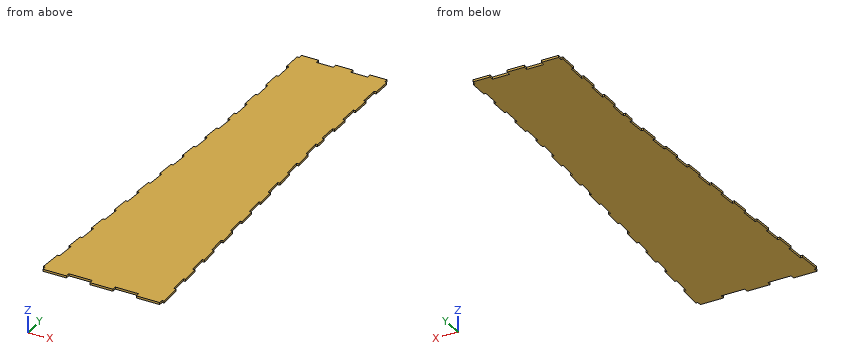
```python
from build123d import *

# Parameters (mm, degrees)
BOSS_EXTRUDE3_DEPTH = 10.16


with BuildPart() as part:
    # Sketch4 → Boss-Extrude3 (new body)
    with BuildSketch(Plane.XY):
        Polygon((-210.367858706, 1373.732193279), (-220.506832234, 1374.260391019), (-225.131875264, 1285.480782003), (-214.992901736, 1284.952584263), (-219.617944766, 1196.172975248), (-229.756918293, 1196.701172988), (-234.381961323, 1107.921563972), (-224.242987795, 1107.393366232), (-228.868030825, 1018.613757216), (-228.874436508, 1018.614090925), (-239.007004353, 1019.141954956), (-243.632047383, 930.362345941), (-233.493073855, 929.834148201), (-238.118116884, 841.054539185), (-248.257090412, 841.582736925), (-252.882133442, 752.803127909), (-242.743159914, 752.274930169), (-247.368202944, 663.495321154), (-247.374608626, 663.495654863), (-257.507176472, 664.023518894), (-262.132219501, 575.243909878), (-251.993245973, 574.715712138), (-256.618289003, 485.936103122), (-266.757262531, 486.464300862), (-271.382305561, 397.684691847), (-261.243332033, 397.156494107), (-265.868375062, 308.376885091), (-276.00734859, 308.905082831), (-280.63239162, 220.125473815), (-270.493418092, 219.597276075), (-275.118461122, 130.81766706), (-285.25743465, 131.3458648), (-291.041413739, 20.32), (-280.874923338, 20.32), (-280.874923338, 0), (-168.302123338, 0), (-168.302123338, 20.32), (-55.729323338, 20.32), (-55.729323338, 0), (55.729323338, 0), (55.729323338, 20.32), (168.302123338, 20.32), (168.302123338, 0), (280.874923338, 0), (280.874923338, 20.32), (291.041413739, 20.32), (285.25743465, 131.3458648), (275.118461122, 130.81766706), (270.493418092, 219.597276075), (280.63239162, 220.125473815), (276.00734859, 308.905082831), (265.868375062, 308.376885091), (261.243332033, 397.156494107), (271.382305561, 397.684691847), (266.757262531, 486.464300862), (256.618289003, 485.936103122), (251.993245973, 574.715712138), (262.132219501, 575.243909878), (257.507176472, 664.023518894), (247.368202944, 663.495321154), (242.743159914, 752.274930169), (252.882133442, 752.803127909), (248.257090412, 841.582736925), (238.118116884, 841.054539185), (233.493073855, 929.834148201), (243.632047383, 930.362345941), (239.007004353, 1019.141954956), (228.868030825, 1018.613757216), (224.242987795, 1107.393366232), (234.381961323, 1107.921563972), (229.756918293, 1196.701172988), (219.617944766, 1196.172975248), (214.992901736, 1284.952584263), (214.999307419, 1284.952917972), (225.131875264, 1285.480782003), (220.506832234, 1374.260391019), (210.367858706, 1373.732193279), (205.715298803, 1463.040000035), (215.881789204, 1463.040000035), (215.881789204, 1518.92), (205.715298803, 1518.92), (205.715298803, 1607.82), (215.881789204, 1607.82), (215.881789204, 1696.72), (205.715298803, 1696.72), (205.715298803, 1785.62), (215.881789204, 1785.62), (215.881789204, 1874.52), (205.715298803, 1874.52), (205.715298803, 1963.42), (215.881789204, 1963.42), (215.881789204, 2052.32), (205.715298803, 2052.32), (205.715298803, 2072.64), (123.444, 2072.64), (123.444, 2052.32), (41.135649402, 2052.32), (41.135649402, 2072.64), (-41.135649402, 2072.64), (-41.135649402, 2052.32), (-123.444, 2052.32), (-123.444, 2072.64), (-205.715298803, 2072.64), (-205.715298803, 2052.32), (-215.881789204, 2052.32), (-215.881789204, 1963.42), (-205.715298803, 1963.42), (-205.715298803, 1874.52), (-215.881789204, 1874.52), (-215.881789204, 1785.62), (-205.715298803, 1785.62), (-205.715298803, 1696.72), (-215.881789204, 1696.72), (-215.881789204, 1607.82), (-205.715298803, 1607.82), (-205.715298803, 1518.92), (-215.881789204, 1518.92), (-215.881789204, 1463.040000035), (-205.715298803, 1463.040000035), align=None)
    extrude(amount=BOSS_EXTRUDE3_DEPTH)


solid = part.part
```
Geometry: final body of the model. Coordinates: model frame, mm. Coordinates: 2 decimals unless noted, no trailing zeros. Write each loop counter-clockwise with the first axis right and the second up, starting at its lowest first coordinate (ties: lowest second). Pieces come first, ordered by that corner, then holes. Notation, with made-up numbers: M 75.25,65 L 79.25,65 A23 ccw 79.25,90 Z; hole C 80.5,71.5 d3. An arc over 180 degrees is marked long. Use CSV: the item, a comma, the result in double quotes. Start each with the question number.
1. Cut plane B-B on x = -99.5. Return the cut outline in (y, z), plus the area to 3 significant figures.
2. First-contact query: P1, Ø5, axis at y = 1833, z = 6, coming from the -X side; P2, Ø5, axis at x = -209, z = 6.5, coming from the +Y side; P3, Ø1, axis at x = -117.5, z = 8.5, coming from the -Y side. Flat tips, straight axial feed; report the tip coordinate or a pass-through.
3. Ray query, probe 1 along X at (y, z) = (1950, 4.5); probe 2 along Y at (x, z) = (-61, 1.5); probe 3 along Y at (x, z) = (-158, 7). Return the intervals inside material, ascending.
4. Cut plane A-A on y = 1487. Return the cut outline in (x, z).
Entries:
1,outline,"M 20.32,0 L 2052.32,0 L 2052.32,10.16 L 20.32,10.16 Z"
1,area,"20,600 mm²"
2,P1,"x = -215.88"
2,P2,"y = 2052.32"
2,P3,"y = 20.32"
3,probe 1,"-205.72 to 205.72"
3,probe 2,"20.32 to 2052.32"
3,probe 3,"20.32 to 2072.64"
4,outline,"M -215.88,0 L 215.88,0 L 215.88,10.16 L -215.88,10.16 Z"
